Verification items for the finished model (mm, model axes). A direction names the side the tool comes from. Round coordinates to 2 decimals unless told otherwise and drop trailing zeros. Order: outer loops, then holes, each group sorted by start corner. A loop starts at its lowest first (then second) coordinate and runs counter-clockwise, first axis right, second up. Notation, with made-up numbers: M 89.25,-36.75 L 132.25,-36.75 A20 cw 132.25,-21.75 Z; hole C 51.25,-11 d3. An arc over 180 degrees is marked long. Use one line per item in the form item = value. Start each with the question number.
Item 1: Go/stop test with flat-tipped pins: pin 1 Ø8 at (x, y) = (19.5, 11) entering from +Z; pin 2 Ø5 at (x, z) = (36, 30.5) entering from -Y. Record where each tip stops, or that it passes through.
Item 2: Tool access check on faces 4 (the flat face through (97, 15, 35)), 5 (the flat face through (49, 20, 10)). Record the directions out of +Z, -Z, +X, -X, +Y, -Y that give a thin tool (end or side, any length) a straight path to the whole face; none if there is none.
Item 3: Cross-section at A-A on x = 72.5. Enter the section's corners in (y, z), then the cut area to 3 significant figures.
Item 4: Cross-section at B-B on y = 20. Enter the section's corners in (x, z), then the cut area to 3 significant figures.
Item 5: Cross-section at D-D on y = 32. Enter the section's corners in (x, z).
Item 6: Release check for a two-part mould opening along Y. For faces 1 (the cylindrical face through (22, 25.1, 5.1)), 2 (the flat face through (5, 24, 25)), 3 (the flat face through (49, 50, 25)) record: +Y half, -Y half, draft (parallel to the pull), parting line (faces both ways), or undercut.
Item 7: Cross-section at C-C on z = 22. Enter the section's corners in (x, y), then the cut area to 3 significant figures.
Item 8: Thickness scan on probe 1 along X at (y, z) = (31.5, 17.5); probe 2 along Y at (x, z) = (27, 8); probe 3 along Y at (x, z) = (5.5, 17). Record the ranges inside material, lowest first. Write a range as [from, to].
from build123d import *

# Parameters (mm, degrees)
F0_W     = 100
F0_H     = 50
F1_DEPTH = 50
F2_T     = -10
F3_R     = 7.5
F4_DEPTH = 10.001
F5_W     = 5
F5_H     = 40
F6_DEPTH = 40
F7_SIZE  = 30


with BuildPart() as f1:
    # F0 (on Top) → F1 (new body)
    with BuildSketch(Plane.XY):
        with Locations((50, 25)):
            Rectangle(F0_W, F0_H)
    extrude(amount=F1_DEPTH)

    # F2
    f2_openings = [f1.faces().sort_by_distance(p)[0] for p in [
        (50, 25, 50),
        (50, 0, 25),
        (100, 25, 25),
        (0, 25, 25),
    ]]
    offset(amount=F2_T, openings=f2_openings)

    # F3 (on face) → F4 (cut, through all)
    with BuildSketch(Plane.XY.offset(10)):
        with Locations((27.5, 20)):
            Circle(F3_R)
        with Locations((72.5, 20)):
            Circle(F3_R)
    extrude(amount=-F4_DEPTH, mode=Mode.SUBTRACT)

    # F5 (on face) → F6 (join)
    with BuildSketch(Plane.XY.offset(10)):
        with Locations((2.5, 20)):
            Rectangle(F5_W, F5_H)
        with Locations((97.5, 20)):
            Rectangle(F5_W, F5_H)
    extrude(amount=F6_DEPTH)

    # F7
    f7_edges = [f1.edges().sort_by_distance(p)[0] for p in [
        (2.5, 0, 50),
        (97.5, 0, 50),
    ]]
    chamfer(f7_edges, length=F7_SIZE)


solid = f1.part
Output values:
q1.pin_1 = 10
q1.pin_2 = 40
q2.face_4 = +Z, +X, -X, -Y
q2.face_5 = +Z, -Y
q3.outline = M 0,0 L 12.5,0 L 12.5,10 L 0,10 Z; M 27.5,0 L 50,0 L 50,50 L 40,50 L 40,10 L 27.5,10 Z
q3.area = 750 mm2
q4.outline = M 0,0 L 20,0 L 20,10 L 5,10 L 5,40 L 0,40 Z; M 35,0 L 65,0 L 65,10 L 35,10 Z; M 80,0 L 100,0 L 100,40 L 95,40 L 95,10 L 80,10 Z
q4.area = 1,000 mm2
q5.outline = M 0,0 L 100,0 L 100,50 L 95,50 L 95,10 L 5,10 L 5,50 L 0,50 Z
q6.face_1 = undercut
q6.face_2 = draft
q6.face_3 = +Y half
q7.outline = M 0,2 L 5,2 L 5,40 L 95,40 L 95,2 L 100,2 L 100,50 L 0,50 Z
q7.area = 1,380 mm2
q8.probe_1 = [0, 5], [95, 100]
q8.probe_2 = [0, 12.52], [27.48, 50]
q8.probe_3 = [40, 50]
